from build123d import *

# Parameters (mm, degrees)
F1_DEPTH    = 5
F4_SIZE     = 2
F5_R        = 5.99999
F6_SIZE     = 4
F7_R        = 10
F8_R        = 8
F9_T1_DEPTH = 22.4376803184
F9_T3_DEPTH = 16.4376803184
F9_T5_DEPTH = 16.4376803184
F10_SIZE    = 2


# Not quite as in the source:
# - a fillet or chamfer that OpenCascade refuses, or shapes differently, is made with other operations: its cross-section is extruded or revolved along the edge and cut away or added
# - a fillet or chamfer is up to 0.001 mm smaller than in the source, because OpenCascade refuses the exact size


with BuildPart() as f1:
    # F0 (on Top) → F1 (new body, symmetric)
    with BuildSketch(Plane.XY):
        with BuildLine():
            ThreePointArc((8.4409715081, -1), (-0.5008703332, -8.4852300446), (-8.5, 0))
            Line((-8.5, 0), (-8.5, 1.5))
            Line((-8.5, 1.5), (-9.5, 1.5))
            Line((-9.5, 1.5), (-11.5, -2.5))
            Line((-11.5, -2.5), (-9.5, -2.5))
            Line((-9.5, -2.5), (-9.5, -10.5))
            Line((-9.5, -10.5), (10.5, -10.5))
            Line((10.5, -10.5), (10.5, 9.5))
            Line((10.5, 9.5), (-13.3090169944, 9.5))
            Line((-13.3090169944, 9.5), (-13.3090169944, -3.5))
            ThreePointArc((-13.3090169944, -3.5), (-17.3090169944, -7.5), (-21.3090169944, -3.5))
            Line((-21.3090169944, -3.5), (-22.3090169944, -3.5))
            Line((-22.3090169944, -3.5), (-22.3090169944, -9.5))
            Line((-22.3090169944, -9.5), (-13.3090169944, -9.5))
            Line((-13.3090169944, -9.5), (-10, -9.5))
            Line((-10, -9.5), (-10, -3))
            Line((-10, -3), (-12.3090169944, -3))
            Line((-12.3090169944, -3), (-9.8090169944, 2))
            Line((-9.8090169944, 2), (-8.2613558209, 2))
            ThreePointArc((-8.2613558209, 2), (0.5080014259, 8.4848060998), (8.4409715081, 1))
            Line((8.4409715081, 1), (10, 1))
            Line((10, 1), (10, -1))
            Line((10, -1), (8.4409715081, -1))
        make_face()
    extrude(amount=F1_DEPTH, both=True)

    # F2 (on Top) → F3 (revolve, cut)
    with BuildSketch(Plane.XY):
        Polygon((0, 0), (-8.5, 0), (-8.5, -3.5), (-2, -10), (-2, -10.5), (0, -10.5), align=None)
    revolve(axis=Axis((0, -4.5, 0), (0, -1, 0)), mode=Mode.SUBTRACT)

    # F4
    f4_edges = [f1.edges().sort_by_distance(p)[0] for p in [
        (-10, -9.5, 0),
    ]]
    chamfer(f4_edges, length=F4_SIZE)

    # F5 (radius 6 in the source; OpenCascade refuses exactly that, so slightly less here)
    f5_edges = [f1.edges().sort_by_distance(p)[0] for p in [
        (-22.309017, -9.5, 0),
    ]]
    fillet(f5_edges, radius=F5_R)

    # F6
    f6_edges = [f1.edges().sort_by_distance(p)[0] for p in [
        (-13.309017, 9.5, 0),
    ]]
    chamfer(f6_edges, length=F6_SIZE)

    # F7
    f7_edges = [f1.edges().sort_by_distance(p)[0] for p in [
        (-9.309017, 9.5, 0),
    ]]
    fillet(f7_edges, radius=F7_R)

    # F8
    f8_edges = [f1.edges().sort_by_distance(p)[0] for p in [
        (-13.309017, 5.5, 0),
    ]]
    fillet(f8_edges, radius=F8_R)

    # F9: fillet of radius 5 on 3 edges, made by hand

    # F9_s2 → F9_t1 (cut)
    with BuildSketch(Plane.XY.offset(-11.2188401592)):
        with BuildLine():
            ThreePointArc((10, 1), (8.693634047, 2.015063424), (7.7900075738, 3.4008501878))
            Line((7.7900075738, 3.4008501878), (7.6983604259, 3.3608401856))
            ThreePointArc((7.6983604259, 3.3608401856), (8.1072760601, 2.1981980996), (8.3416659609, 0.9882352941))
            Line((8.3416659609, 0.9882352941), (8.4409715081, 0.9))
            ThreePointArc((8.4409715081, 0.9), (9.220485754, 0.9), (9.9525527006, 0.911972994))
            Line((9.9525527006, 0.911972994), (10, 1))
        make_face()
    extrude(amount=F9_T1_DEPTH, mode=Mode.SUBTRACT)

    # F9_s4 → F9_t3 (cut)
    with BuildSketch(Plane.XY.offset(-11.2188401592)):
        with BuildLine():
            ThreePointArc((7.7900075738, -3.4008501878), (8.693634047, -2.015063424), (10, -1))
            Line((10, -1), (9.9525527006, -0.911972994))
            ThreePointArc((9.9525527006, -0.911972994), (9.220485754, -0.9), (8.4409715081, -0.9))
            Line((8.4409715081, -0.9), (8.3416659609, -0.9882352941))
            ThreePointArc((8.3416659609, -0.9882352941), (8.1072760601, -2.1981980996), (7.6983604259, -3.3608401856))
            Line((7.6983604259, -3.3608401856), (7.7900075738, -3.4008501878))
        make_face()
    extrude(amount=F9_T3_DEPTH, mode=Mode.SUBTRACT)

    # F9_s6 → F9_t5 (cut)
    with BuildSketch(Plane.XY.offset(-5.2188401592)):
        with BuildLine():
            ThreePointArc((7.7900075738, -3.4008501878), (8.693634047, -2.015063424), (10, -1))
            Line((10, -1), (9.9525527006, -0.911972994))
            ThreePointArc((9.9525527006, -0.911972994), (9.220485754, -0.9), (8.4409715081, -0.9))
            Line((8.4409715081, -0.9), (8.3416659609, -0.9882352941))
            ThreePointArc((8.3416659609, -0.9882352941), (8.1072760601, -2.1981980996), (7.6983604259, -3.3608401856))
            Line((7.6983604259, -3.3608401856), (7.7900075738, -3.4008501878))
        make_face()
    extrude(amount=F9_T5_DEPTH, mode=Mode.SUBTRACT)

    # F10
    f10_edges = [f1.edges().sort_by_distance(p)[0] for p in [
        (10.5, 9.5, 0),
    ]]
    chamfer(f10_edges, length=F10_SIZE)


solid = f1.part
Build history of the part. All positions in model axes, mm. A direction names the side the tool comes from. Give positions to 0.01 mm unless a question says otherwise; leave off trailing zeros. Write each loop counter-clockwise with the first axis right and the second up, starting at its lowest first coordinate (ties: lowest second). Pieces come first, ordered by that corner, then holes. Notation, with made-up numbers: (78, -24.75) - (82, -24.75) arc R34 cw to (82, 8.25) - close; hole circle Ø9 at (19, 72). An arc over 180 degrees is marked (long way). Use one line per item in the form item = value. Start each with the question number.
1. Band-saw the part on D-D on x = -17.5. Write the cut outline in (y, z), plus the area to 3 significant figures.
2. Band-saw the part on C-C on x = -11. Count the separate pieces of the cut face and the enclosed holes in it, plus the area to 3 significant figures.
3. Band-saw the part on A-A on x = 0. Write the cut outline in (y, z).
4. Band-saw the part on B-B on y = -4.5. Write the cut outline in (x, z), plus the area to 3 significant figures.
5. Two-plate mould, pull along Z, no slides. Class faces 1 (the face through (-6, -6.4, -5)), 2 (the face through (8.71, 2, -0.07)), 3 (the face through (-6, -6.4, 5)), 4 (the face through (8.5, -3, -0.1)): released by +Z, released by -Z, zero draft, split by the parting line, or undercut.
6. Probe line 1 (Z direction, x = 0, y = -10.4); line 2 (X direction, y = -10.3, z = 0); line 3 (Y direction, x = -3.5, z = 4.5). List the from-to ranges inside material, lowest first. Write a range as [from, to].
7. Drop flat-ended pins along their axis: pin 1 Ø4 at (y, z) = (-6.5, -1.5) entering from -X; pin 2 Ø1.6 at (x, z) = (-10.5, -1.5) entering from -Y; pin 3 Ø1 at (y, z) = (-0.5, 0) entering from -X. Give the stop position or say it passes through.
8. 3-axis set-ups, long thin cutter, end or side, ignore diameter. For faces 5 (the face through (-14, -9.5, 0)), 6 (the face through (-22, -3.5, 0)), 7 (the face through (-8, -4, 0)), 8 (the face through (-0.887, 8.454, 0.07)): which of +Z, -Z, +X, -X, +Y, -Y reach the whole face in a straight line?
Conclusion:
q1.outline = (-9.38, -5) - (-7.5, -5) - (-7.5, 5) - (-9.38, 5) - close
q1.area = 18.9 mm²
q2.separate_pieces = 3
q2.enclosed_holes = 0
q2.area = 140 mm²
q3.outline = (-10.5, -5) - (-8.5, -5) - (-8.5, -3.5) - (-10, -2) - (-10.5, -2) - close; (-10.5, 2) - (-10, 2) - (-8.5, 3.5) - (-8.5, 5) - (-10.5, 5) - close; (8.5, -5) - (9.5, -5) - (9.5, 5) - (8.5, 5) - close
q4.outline = (-22.23, -5) - (-21.18, -5) - (-21.18, 5) - (-22.23, 5) - close; (-13.44, -5) - (-10, -5) - (-10, 5) - (-13.44, 5) - close; (-9.5, -5) - (-7.21, -5) - (-7.21, -2.06) arc R7.5 cw to (-7.21, 2.06) - (-7.21, 5) - (-9.5, 5) - close; (7.21, -5) - (10.5, -5) - (10.5, 5) - (7.21, 5) - (7.21, 2.06) arc R7.5 cw to (7.21, -2.06) - close
q4.area = 99.0 mm²
q5.face_1 = released by -Z
q5.face_2 = zero draft
q5.face_3 = released by +Z
q5.face_4 = undercut
q6.line_1 = [-5, -2], [2, 5]
q6.line_2 = [-9.5, -2], [2, 10.5]
q6.line_3 = [-10.5, -7.75], [7.75, 9.5]
q7.pin_1 = -22.23
q7.pin_2 = -8.8
q7.pin_3 = -13.31
q8.face_5 = +Z, -Z, -X, -Y
q8.face_6 = +Z, -Z, -X, +Y
q8.face_7 = none
q8.face_8 = +Z, -Z
